from build123d import *

# Parameters (mm, degrees)
BOSS_EXTRUDE1_DEPTH = 6
SKETCH2_W           = 21.1
SKETCH2_H           = 15.1
BOSS_EXTRUDE2_DEPTH = 2
FILLET1_R           = 1
SKETCH3_R           = 0.816975511
BOSS_EXTRUDE3_DEPTH = 0.85
LPATTERN1_COUNT     = 2
LPATTERN1_PITCH     = 6
BOSS_EXTRUDE4_DEPTH = 4.75
BOSS_EXTRUDE5_DEPTH = 2.5


with BuildPart() as part:
    # Sketch1 → Boss-Extrude1 (new, symmetric)
    with BuildSketch(Plane(origin=(0, 0, 0), x_dir=(1, 0, 0), z_dir=(0, 1, 0))):
        Polygon((-8.3, 0), (8.3, 0), (8.3, -1), (9.4, -1), (9.4, 2.2), (8.8, 2.2), (8.8, 10.5), (-8.8, 10.5), (-8.8, 2.2), (-9.4, 2.2), (-9.4, -1), (-8.3, -1), align=None)
    extrude(amount=BOSS_EXTRUDE1_DEPTH, both=True)

    # Sketch2 → Boss-Extrude2 (add)
    with BuildSketch(Plane(origin=(0, 0, -10.5), x_dir=(-1, 0, 0), z_dir=(0, 0, -1))):
        Rectangle(SKETCH2_W, SKETCH2_H)
    extrude(amount=BOSS_EXTRUDE2_DEPTH)

    # Fillet1
    fillet1_edges = [part.edges().sort_by_distance(p)[0] for p in [
        (10.55, 7.55, -11.5),
        (10.55, -7.55, -11.5),
        (-10.55, -7.55, -11.5),
        (-10.55, 7.55, -11.5),
    ]]
    fillet(fillet1_edges, radius=FILLET1_R)

    # Sketch3 → Boss-Extrude3 (add, symmetric)
    with BuildSketch(Plane(origin=(0, 0, 0), x_dir=(0, 0, -1), z_dir=(1, 0, 0))):
        Polygon((0, 2.5), (-6.8, 2.5), (-7.8, 1.5), (-7.8, -1.5), (-6.8, -2.5), (0, -2.5), align=None)
        with Locations((-4.630991461, 0)):
            Circle(SKETCH3_R, mode=Mode.SUBTRACT)
    boss_extrude3 = extrude(amount=BOSS_EXTRUDE3_DEPTH, both=True)

    # LPattern1: Boss-Extrude3 ×2
    with Locations(*[(i * LPATTERN1_PITCH, 0, 0) for i in range(1, LPATTERN1_COUNT)]):
        add(boss_extrude3)

    # Sketch4 → Boss-Extrude4 (add, symmetric)
    with BuildSketch(Plane(origin=(0, 0, 0), x_dir=(1, 0, 0), z_dir=(0, 1, 0))):
        with BuildLine():
            Line((7.176954922, 12.800602649), (7.176954922, 12.5))
            Line((7.176954922, 12.5), (-7.71090433, 12.5))
            ThreePointArc((-7.71090433, 12.5), (-6.700290902, 15.093362546), (-5.21395506, 17.446588959))
            ThreePointArc((-5.21395506, 17.446588959), (-4.414402061, 17.834047388), (-3.622018998, 17.432129346))
            ThreePointArc((-3.622018998, 17.432129346), (1.155737297, 13.666724512), (7.176954922, 12.800602649))
        make_face()
    extrude(amount=BOSS_EXTRUDE4_DEPTH, both=True)

    # Sketch5 → Boss-Extrude5 (add, symmetric)
    with BuildSketch(Plane(origin=(0, 0, 0), x_dir=(1, 0, 0), z_dir=(0, 1, 0))):
        Polygon((8.8, 10.5), (9.730151973, 6.35), (8.8, 2.2), (9.619848027, 2.2), (10.55, 6.35), (9.619848027, 10.5), align=None)
    boss_extrude5 = extrude(amount=BOSS_EXTRUDE5_DEPTH, both=True)

    # Mirror1: Boss-Extrude5 across plane
    add(boss_extrude5.mirror(Plane(origin=(0, 0, 0), x_dir=(0, 0, 1), z_dir=(1, 0, 0))))


solid = part.part
Read the model definition and answer for the solid it produces. Units are mm, in the model's axes. A direction names the side the tool comes from. Round coordinates to 2 decimals unless told otherwise and drop trailing zeros. Write each loop counter-clockwise with the first axis right and the second up, starting at its lowest first coordinate (ties: lowest second). Pieces come first, ordered by that corner, then holes.
1. Straight lines are drawn through the part: L1, parallel to X at y = 0.75, z = 3; L2, parallel to X at y = 1, z = -4.5; L3, parallel to Y at x = 8.75, z = -1.75. For each, find the intervals that lie inside material, in ascending order.
2. Given pin 1 Ø3.5 at (x, z) = (2, -4) entering from -Y; pin 2 Ø6 at (x, y) = (0.5, 3.5) entering from -Z; pin 3 Ø1 at (x, z) = (5, -2.5) entering from +Y, each flat-ended and moving along its own axis, determine where each tip first touches the part or whether it passes through.
3. The part is cut by section A-A, the plane z = 6. Determine the outline of the cut face in (x, y), then the cut area to 3 significant figures.
4. Determine the mould class of faces 1 (the face through (10.09, 0.04, -8.4)), 2 (the face through (-9, 0, 1)), 3 (the face through (-6.718, 0.067, -15.058)) for opening direction Z: pulls with the +Z half, pulls with the -Z half, needs draft (parallel to the pull), parting line crosses it, or undercut.
5. Which of the six approach directions +Z, -Z, +X, -X, +Y, -Y give full straight-line access (tool end or side, diameter ignored) to faces 4 (the face through (0, -6, -5)), 5 (the face through (8.3, 0.1, 0.5)), 6 (the face through (10.08, 0.04, -4.25)), 7 (the face through (10, -2.5, -6))?
6. The part is cut by section B-B, the plane y = 0. State how many separate pieces and enclosed holes the cut face has, then the cut area to 3 significant figures.
7. The part is cut by section C-C, the plane x = -2.75. Determine the outline of the cut face in (y, z).
Values:
1. L1: x = -0.85 to 0.85, 5.15 to 6.85
1. L2: x = -10.14 to -9.32, -8.8 to 8.8, 9.32 to 10.14
1. L3: y = -6 to 6
2. pin 1: stops at y = -6
2. pin 2: stops at z = -16.14
2. pin 3: stops at y = 6
3. outline: (-0.85, -2.5) - (0.85, -2.5) - (0.85, 2.5) - (-0.85, 2.5) - close; (5.15, -2.5) - (6.85, -2.5) - (6.85, 2.5) - (5.15, 2.5) - close
3. area: 17.0 mm2
4. face 1: undercut
4. face 2: pulls with the +Z half
4. face 3: pulls with the -Z half
5. face 4: +Z, +X, -X, -Y
5. face 5: +Z, +Y, -Y
5. face 6: +Z, +X, +Y, -Y
5. face 7: +X, -Y
6. separate pieces: 3
6. enclosed holes: 2
6. area: 298 mm2
7. outline: (-7.55, -12.5) - (-4.75, -12.5) - (-4.75, -16.39) - (4.75, -16.39) - (4.75, -12.5) - (7.55, -12.5) - (7.55, -10.5) - (6, -10.5) - (6, 0) - (-6, 0) - (-6, -10.5) - (-7.55, -10.5) - close
